Verification items for the finished model (mm, model axes). Give positions to 0.01 mm unless a question says otherwise; leave off trailing zeros. Write each loop counter-clockwise with the first axis right and the second up, starting at its lowest first coordinate (ties: lowest second). Pieces come first, ordered by that corner, then holes. Notation, with made-up numbers: (-20, 7) -> (-9, 7) arc R14 cw to (-9, 23) -> close; hole circle Ø7 at (74.25, 86.5). An arc over 180 degrees is marked (long way). Use CSV: the item, a comma, the result in double quotes. Start each with the question number.
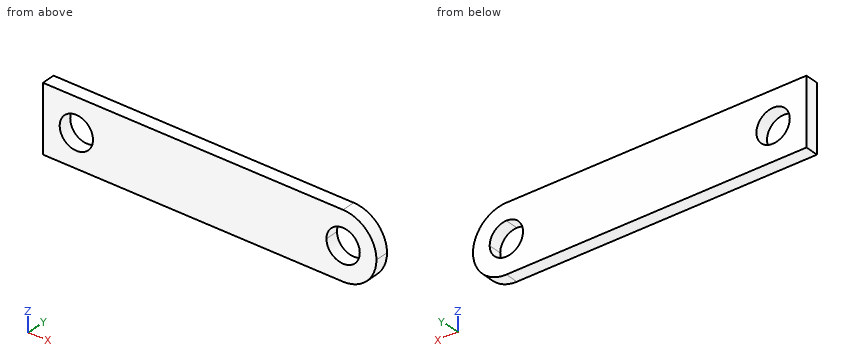
```python
from build123d import *

# Parameters (mm, degrees)
SALIENTE_EXTRUIR2_DEPTH   = 2
SALIENTE_EXTRUIR2_2_DEPTH = 2
SALIENTE_EXTRUIR5_DEPTH   = 2


with BuildPart() as part:
    # Croquis1 → Saliente-Extruir2 (new body)
    with BuildSketch(Plane(origin=(0, 0, 0), x_dir=(1, 0, 0), z_dir=(0, 1, 0))):
        with BuildLine():
            Line((25, 0), (27.5, 0))
            ThreePointArc((27.5, 0), (22.5, 5), (17.5, 0))
            Line((17.5, 0), (20, 0))
            ThreePointArc((20, 0), (22.5, 2.5), (25, 0))
        make_face()
    extrude(amount=SALIENTE_EXTRUIR2_DEPTH)



with BuildPart() as body_2:
    # Croquis1 → Saliente-Extruir2 2 (new body)
    with BuildSketch(Plane(origin=(0, 0, 0), x_dir=(1, 0, 0), z_dir=(0, 1, 0))):
        with BuildLine():
            Line((-22.5, -5), (22.5, -5))
            ThreePointArc((22.5, -5), (18.964466094, -3.535533906), (17.5, 0))
            Line((17.5, 0), (-15, 0))
            ThreePointArc((-15, 0), (-17.5, -2.5), (-20, 0))
            Line((-20, 0), (-22.5, 0))
            Line((-22.5, 0), (-22.5, -5))
        make_face()
    extrude(amount=SALIENTE_EXTRUIR2_2_DEPTH)


with BuildPart() as part_1:
    add(part.part)

    add(body_2.part)  # Saliente-Extruir5 merges body 2
    # Croquis1_4 → Saliente-Extruir5 (add)
    with BuildSketch(Plane(origin=(0, 0, 0), x_dir=(1, 0, 0), z_dir=(0, 1, 0))):
        with BuildLine():
            ThreePointArc((17.5, 0), (18.964466094, 3.535533906), (22.5, 5))
            Line((22.5, 5), (-22.5, 5))
            Line((-22.5, 5), (-22.5, 0))
            Line((-22.5, 0), (-20, 0))
            ThreePointArc((-20, 0), (-17.5, 2.5), (-15, 0))
            Line((-15, 0), (17.5, 0))
        make_face()
        with BuildLine():
            ThreePointArc((22.5, 2.5), (24.267766953, 1.767766953), (25, 0))
            Line((25, 0), (27.5, 0))
            ThreePointArc((27.5, 0), (26.035533906, 3.535533906), (22.5, 5))
            Line((22.5, 5), (22.5, 2.5))
        make_face()
        with BuildLine():
            Line((27.5, 0), (25, 0))
            ThreePointArc((25, 0), (24.267766953, -1.767766953), (22.5, -2.5))
            Line((22.5, -2.5), (22.5, -5))
            ThreePointArc((22.5, -5), (26.035533906, -3.535533906), (27.5, 0))
        make_face()
        with BuildLine():
            ThreePointArc((20, 0), (20.732233047, 1.767766953), (22.5, 2.5))
            Line((22.5, 2.5), (22.5, 5))
            ThreePointArc((22.5, 5), (18.964466094, 3.535533906), (17.5, 0))
            Line((17.5, 0), (20, 0))
        make_face()
        with BuildLine():
            Line((22.5, -5), (22.5, -2.5))
            ThreePointArc((22.5, -2.5), (20.732233047, -1.767766953), (20, 0))
            Line((20, 0), (17.5, 0))
            ThreePointArc((17.5, 0), (18.964466094, -3.535533906), (22.5, -5))
        make_face()
    extrude(amount=SALIENTE_EXTRUIR5_DEPTH)


solid = part_1.part
```
(1) Section check D-D on z = -3.25. Record the cut outline in (x, y), then the cut area to 3 significant figures.
(2) Thickness scan on line 1 (Z direction, x = -17.5, y = 0.7); line 2 (X direction, y = 1.6, z = -2); line 3 (X direction, y = 1.1, z = -0.5). Record the ranges inside material, lowest first. Write a range as from..to.
(3) Section check A-A on y = 0.3. Record the cut outline in (x, z).
(4) Section check B-B on x = -17.5. Record the cut outline in (y, z), then the cut area to 3 significant figures.
(5) Section check C-C on z = -0.75. Record the cut outline in (x, y), then the cut area to 3 significant figures.
Data:
1,outline,"(-22.5, 0) -> (26.3, 0) -> (26.3, 2) -> (-22.5, 2) -> close"
1,area,"97.6 mm2"
2,line 1,"z = -5..-2.5, 2.5..5"
2,line 2,"x = -22.5..-19, -16..21, 24..27.08"
2,line 3,"x = -22.5..-19.95, -15.05..20.05, 24.95..27.47"
3,outline,"(-22.5, -5) -> (22.5, -5) arc R5 ccw to (22.5, 5) -> (-22.5, 5) -> close; hole circle Ø5 at (-17.5, 0); hole circle Ø5 at (22.5, 0)"
4,outline,"(0, -5) -> (2, -5) -> (2, -2.5) -> (0, -2.5) -> close; (0, 2.5) -> (2, 2.5) -> (2, 5) -> (0, 5) -> close"
4,area,"10.0 mm2"
5,outline,"(-22.5, 0) -> (-19.88, 0) -> (-19.88, 2) -> (-22.5, 2) -> close; (-15.12, 0) -> (20.12, 0) -> (20.12, 2) -> (-15.12, 2) -> close; (24.88, 0) -> (27.44, 0) -> (27.44, 2) -> (24.88, 2) -> close"
5,area,"80.8 mm2"
